Can you work these out from the drawing? Everything is in mm from the part's minimum corner. Coordinates: 2 decimals unless noted, no trailing zeros. Loops run counter-clockwise (first coordinate to the right, second up) from the corner with the lowest first, then second, coordinate; pieces in that order, holes last. Notation, with made-up numbers: (48.25, 62) -> (65.25, 62) arc R23 cw to (65.25, 101) -> close; hole circle Ø3 at (69, 78). An arc over 180 degrees is marked (long way). Put each result on its own line as item: value. Start each with the question number.
Item 1: Please list where these lines run through material, in increasing order: L1, parallel to Y at x = 129, z = 879.5; L2, parallel to Y at x = 906.5, z = 937; L3, parallel to X at y = 957.5, z = 563.5. Write a range as from..to.
Item 2: If we section it at C-C on x = 244: Please give me the cut outline in (y, z).
Item 3: If we section it at D-D on z = 345.5: Please give me the cut outline in (x, y), plus the area to 3 significant figures.
Item 4: If we section it at B-B on z = 914.5: Please give me the cut outline in (x, y).
Item 5: Will these pins go through, and if not, where does the flat tip stop? P1, Ø2, axis at x = 445, y = 553.5, coming from the +Z side; P2, Ø5, axis at x = 141, y = 414.5, coming from the +Z side; P3, Ø5, axis at x = 209.5, z = 323, coming from the -Y side.
Item 6: If we section it at A-A on y = 545: Please give me the cut outline in (x, z), plus the area to 3 significant figures.
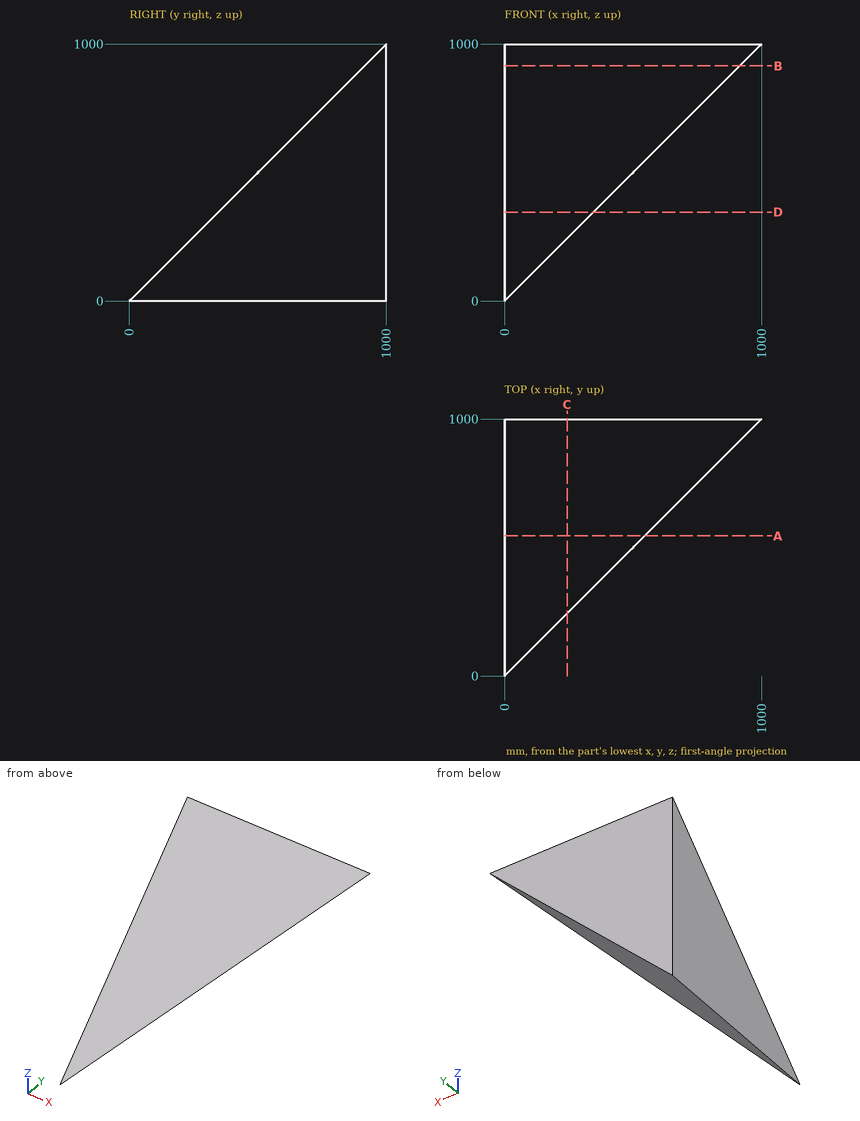
Solutions:
1. L1: 879.5..1000
1. L2: 937..1000
1. L3: 0..563.5
2. outline: (244, 244) -> (1000, 244) -> (1000, 1000) -> close
3. outline: (0, 345.5) -> (345.5, 345.5) -> (345.5, 1000) -> (0, 1000) -> close
3. area: 226,000 mm^2
4. outline: (0, 914.5) -> (914.5, 914.5) -> (914.5, 1000) -> (0, 1000) -> close
5. P1: z = 554.5
5. P2: z = 417
5. P3: y = 320.5
6. outline: (0, 0) -> (545, 545) -> (0, 545) -> close
6. area: 149,000 mm^2
